```python
from build123d import *

# Parameters (mm, degrees)
CONG_1_R = 10


with BuildPart() as part:
    # Esquisse1 → Révolution1 (revolve)
    with BuildSketch(Plane.XY, mode=Mode.PRIVATE) as r_volution1_sk:
        Polygon((0, -3.3), (8.21555598, -3.3), (12.5, -0.3), (12.5, 0), (0, 0), align=None)
    revolve(r_volution1_sk.sketch.rotate(Axis((0, 0, 0), (0, -1, 0)), 180), axis=Axis((0, 0, 0), (0, -1, 0)))

    # Congé1
    cong_1_edges = [part.edges().sort_by_distance(p)[0] for p in [
        (8.21555598, -3.3, 0),
    ]]
    fillet(cong_1_edges, radius=CONG_1_R)

    # Esquisse2 → Fraisage pour vis à tête fraisée M31 (revolve, cut)
    with BuildSketch(Plane(origin=(0, -3.3, 0), x_dir=(0, 0, -1), z_dir=(1, 0, 0))):
        Polygon((0, 0), (0, 3.3), (1.7, 3.3), (1.7, 1.8), (3.5, 0), align=None)
    revolve(axis=Axis((0, -9.65, 0), (0, 1, 0)), mode=Mode.SUBTRACT)


solid = part.part
```
Can you work these out from the model? Positions are in its coordinate system, mm. Round coordinates to 2 decimals unless told otherwise and drop trailing zeros. Answer in a Markdown table with one row per item.
Item 1: If I drill on probe 1 along Z at (x, y) = (1.25, -2); probe 2 along Y at (x, z) = (5.5, -10.5); probe 3 along Y at (x, z) = (2.5, 8.5), over which ranges is the centre line in solid material (lowest first)?
Answer block:
| item | result |
|---|---|
| probe 1 | -9.91 to -1.81, 1.81 to 9.91 |
| probe 2 | -0.75 to 0 |
| probe 3 | -2.55 to 0 |
Item 2: We'd pull the mould along Z, two halves only. Please class faces 1 (the cylindrical face through (-5.77, -0.15, 11.09)), 2 (the cylindrical face through (1.66, -0.76, 0.37)), 3 (the flat face through (0, 0, 3)): released by +Z, released by -Z, zero draft, split by the parting line, or undercut.
Answer block:
| item | result |
|---|---|
| face 1 | split by the parting line |
| face 2 | undercut |
| face 3 | zero draft |
Item 3: Will these pins go through, and if not, where does the flat tip stop? P1, Ø1.5, axis at x = -4.5, y = -0.5, coming from the +Z side; P2, Ø3, axis at x = 0, z = 0, coming from the -Y side; P3, Ø1, axis at x = -5.5, y = -1.5, coming from the +Z side.
Answer block:
| item | result |
|---|---|
| P1 | z = 11.92 |
| P2 | through |
| P3 | z = 10.14 |
